from build123d import *

# Parameters (mm, degrees)
SKETCH_1_R               = 10
EXTRUDE_1_DEPTH          = 3
EXTRUDE_1_TAPER          = 35
SKETCH_2_W               = 4
SKETCH_2_H               = 20
EXTRUDE_2_DEPTH          = 2
PATTERN_CIRCULAR_1_COUNT = 8


with BuildPart() as part:
    # Эскиз1 → Бобышка-Вытянуть1 (new body)
    with BuildSketch(Plane(origin=(0, 0, 0), x_dir=(1, 0, 0), z_dir=(0, 1, 0))):
        Circle(SKETCH_1_R)
    extrude(amount=EXTRUDE_1_DEPTH, taper=EXTRUDE_1_TAPER)

    # Эскиз2 → Бобышка-Вытянуть2 (add)
    with BuildSketch(Plane.XZ):
        with Locations((0, 17)):
            Rectangle(SKETCH_2_W, SKETCH_2_H)
    extrude_2 = extrude(amount=-EXTRUDE_2_DEPTH)

    # Круговой массив1: Бобышка-Вытянуть2 ×8 about axis
    pattern_circular_1_axis = Axis((0, 0, 0), (0, 1, 0))
    for i in range(1, PATTERN_CIRCULAR_1_COUNT):
        add(extrude_2.rotate(pattern_circular_1_axis, i * 360 / PATTERN_CIRCULAR_1_COUNT))


solid = part.part
The listing builds one solid part. Answer for the finished solid, in the listing's coordinates (mm). A direction names the side the tool comes from. Give positions to 0.01 mm unless a question says otherwise; leave off trailing zeros. Write each loop counter-clockwise with the first axis right and the second up, starting at its lowest first coordinate (ties: lowest second). Pieces come first, ordered by that corner, then holes. Notation, with made-up numbers: (38.5, 28) - (78.5, 28) arc R17 cw to (78.5, 37) - close; hole circle Ø11 at (26, -2.75). An arc over 180 degrees is marked (long way). Use a Markdown table: item, result.
1. For a pull along Z with two mould halves and no side action, classify faces 4 (the flat face through (-19.112, 0.986, 19.072)), 5 (the flat face through (27, 1, 0)), 6 (the flat face through (-10.997, 0.986, -13.825)), 7 (the flat face through (18, 1, 2)) as released by +Z, released by -Z, zero draft, split by the parting line, or undercut.
Values follow:
| item | result |
|---|---|
| face 4 | released by +Z |
| face 5 | zero draft |
| face 6 | released by -Z |
| face 7 | undercut |
2. Each of these flat-tipped pins is pushed along its axis until it touches: P1, Ø1, axis at y = 1, z = 18.5, coming from the -X side; P2, Ø8, axis at x = 11.5, z = 12.5, coming from the +Y side; P3, Ø13, axis at x = -10, z = -10.5, coming from the +Y side. Where does it stop, or does it pass through?
Values follow:
| item | result |
|---|---|
| P1 | stops at x = -20.18 |
| P2 | stops at y = 2 |
| P3 | stops at y = 2.86 |
3. Section C-C on z = -23 is taken. Write down the section's boundary in (x, y), plus the area to 3 significant figures.
Values follow:
| item | result |
|---|---|
| outline | (-2, 0) - (2, 0) - (2, 2) - (-2, 2) - close |
| area | 8.00 mm² |
4. A tool of negligible diameter and unlimited length cuts with its end or side. For faces 1 (the flat face through (13, 2, 13)), 2 (the flat face through (-27, 1, 0)), 3 (the flat face through (0, 2, -18)), from which of +Z, -Z, +X, -X, +Y, -Y can it reach the whole face along a straight path? Write none if from no direction.
Values follow:
| item | result |
|---|---|
| face 1 | +Z, +X, +Y |
| face 2 | +Z, -Z, -X, +Y, -Y |
| face 3 | -Z, +X, -X, +Y |
5. Find the intervals of material crossed by probe 1 along Z at (x, y) = (-16, 1.25); probe 2 along Z at (x, y) = (10, 1.6); probe 3 along X at (y, z) = (0.6, -19), in increasing order. Write a range as from..to.
Values follow:
| item | result |
|---|---|
| probe 1 | z = -18.83..-13.17, -2..2, 13.17..18.83 |
| probe 2 | z = -12.83..-7.17, -2..2, 7.17..12.83 |
| probe 3 | x = -19.18..-16.17, -2..2, 16.17..19.18 |
6. Section A-A on x = -12 is taken. Write down the section's boundary in (y, z).
Values follow:
| item | result |
|---|---|
| outline | (0, -14.83) - (2, -14.83) - (2, -9.17) - (0, -9.17) - close; (0, -2) - (2, -2) - (2, 2) - (0, 2) - close; (0, 9.17) - (2, 9.17) - (2, 14.83) - (0, 14.83) - close |
7. Section D-D on x = 0 is taken. Write down the section's boundary in (y, z), plus the area to 3 significant figures.
Values follow:
| item | result |
|---|---|
| outline | (0, -27) - (2, -27) - (2, -8.6) - (3, -7.9) - (3, 7.9) - (2, 8.6) - (2, 27) - (0, 27) - close |
| area | 124 mm² |
